Autodesk Inventor part; units mm, degrees
ref_plane "YZ Plane" through (0, 0, 0) normal (1, 0, 0) x (0, 1, 0)
ref_plane "XY Plane" through (0, 0, 0) normal (0, 0, 1) x (1, 0, 0)
sketch "スケッチ1" plane through (0, 0, 0) normal (0, 1, 0) x (-1, 0, 0)
  line L0 (6.5, -6.5) -> (-6.5, -6.5)
  line L1 (-6.5, -6.5) -> (-6.5, 6.5)
  line L2 (-6.5, 6.5) -> (6.5, 6.5)
  line L3 (6.5, 6.5) -> (6.5, -6.5)
  line L4 (6.5, -6.5) -> (-6.5, 6.5) construction
  line L5 (-6.5, -6.5) -> (6.5, 6.5) construction
  dimension "d1" = 13
  dimension "d2" = 13
extrude "押し出し4" add sketch "スケッチ1" along normal blind 5
ref_plane "作業平面2" through (0, 5, 0) normal (0, 1, 0) x (-1, 0, 0)
sketch "スケッチ3" plane through (0, 5, 0) normal (0, 1, 0) x (-1, 0, 0)
  line L0 (4, -4) -> (-4, -4)
  line L1 (-4, -4) -> (-4, 4)
  line L2 (-4, 4) -> (4, 4)
  line L3 (4, 4) -> (4, -4)
  line L4 (4, -4) -> (-4, 4) construction
  line L5 (-4, -4) -> (4, 4) construction
  line L6 (5, -5) -> (-5, -5)
  line L7 (-5, -5) -> (-5, 5)
  line L8 (-5, 5) -> (5, 5)
  line L9 (5, 5) -> (5, -5)
  line L10 (5, -5) -> (-5, 5) construction
  line L11 (-5, -5) -> (5, 5) construction
  point P0 (0, 0)
  point P1 (0, 0)
  dimension "d19" = 8
  dimension "d20" = 8
  dimension "d21" = 10
  dimension "d22" = 10
extrude "押し出し5" cut sketch "スケッチ3" against normal blind 3
hole "穴1" at (0, 5, 0) direction (0, -1, 0) diameter 3.242 end through all
fillet "フィレット1" radius 1 4 edges at (0, 0, -6.5) (6.5, 0, 0) (-6.5, 0, 0) (0, 0, 6.5)
sketch "スケッチ4" plane through (0, 5, 0) normal (0, 1, 0) x (1, 0, 0)
  point P0 (0, 0)
sketch "スケッチ5" plane through (0, 5, 0) normal (0, 1, 0) x (1, 0, 0)
  point P0 (0, 0)
properties part number "pin_joint_ver1"
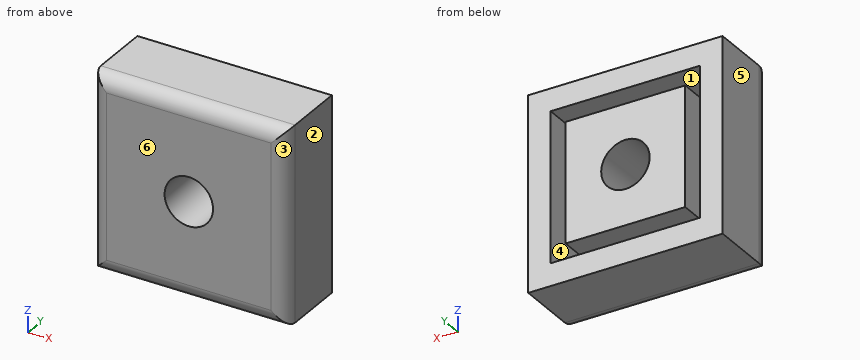
Could you check a few things on this model? Use its own coordinates, in mm. Face numbers are marked on the shaded views. A direction names the side the tool comes from. Give positions to 0.01 mm unless a question says otherwise; leave off trailing zeros. Order: outer loops, then holes, each group sorted by start corner. A loop starts at its lowest first (then second) coordinate and runs counter-clockwise, first axis right, second up. Notation, with made-up numbers: (65, 89.5) -> (104, 89.5) arc R23 cw to (104, 121.5) -> close; hole circle Ø2 at (-24, -9). An arc over 180 degrees is marked (long way). Answer in a Markdown table with one row per item. Add a question column.
Item 1: We'd pull the mould along X, two halves only. Please class the marked faces 3, 4, 5 and 6: pulls with the +X half, pulls with the -X half, needs draft (parallel to the pull), parting line crosses it, or undercut.
Item 2: I'm going to push a flat-ended pin straight in: P1, Ø3, axis at y = 0.5, z = 4, coming from the -X side. Where does the tip first touch, or does it pass through?
Item 3: Please list where these lines run through material, in increasing order: probe 1 along Z at (x, y) = (0, 3.1); probe 2 along X at (y, z) = (3.95, -2.25).
Item 4: Imagine slicing it at D-D (z = 3). List the corners of the cut face in (x, y) for me.
Item 5: Imagine slicing it at A-A (y = 3.4). List the corners of the cut face in (x, z) for me, and give its area (3 significant figures).
Item 6: For the marked faces 1 and 2, which set-ups out of +Z, -Z, +X, -X, +Y, -Y let a thin tool reach every point of the face, with its end or its side?
Item 7: Imagine slicing it at C-C (z = 0). List the corners of the cut face in (x, y) for me.
Item 8: Imagine slicing it at B-B (x = 0). List the corners of the cut face in (y, z) for me.
Result:
| question | item | result |
|---|---|---|
| 1 | face 3 | pulls with the +X half |
| 1 | face 4 | undercut |
| 1 | face 5 | pulls with the -X half |
| 1 | face 6 | needs draft |
| 2 | P1 | x = -6.5 |
| 3 | probe 1 | -6.5 to -5, -4 to -1.62, 1.62 to 4, 5 to 6.5 |
| 3 | probe 2 | -6.5 to -5, -4 to 4, 5 to 6.5 |
| 4 | outline | (-6.5, 1) arc R1 ccw to (-5.5, 0) -> (5.5, 0) arc R1 ccw to (6.5, 1) -> (6.5, 5) -> (5, 5) -> (5, 2) -> (4, 2) -> (4, 5) -> (-4, 5) -> (-4, 2) -> (-5, 2) -> (-5, 5) -> (-6.5, 5) -> close |
| 5 | outline | (-6.5, -6.5) -> (6.5, -6.5) -> (6.5, 6.5) -> (-6.5, 6.5) -> close; (-4, -4) -> (4, -4) -> (4, 4) -> (-4, 4) -> close; hole (-5, -5) -> (5, -5) -> (5, 5) -> (-5, 5) -> close; hole circle Ø3.24 at (0, 0) |
| 5 | area | 125 mm2 |
| 6 | face 1 | +Y |
| 6 | face 2 | +Z, -Z, +X, +Y, -Y |
| 7 | outline | (-6.5, 1) arc R1 ccw to (-5.5, 0) -> (-1.62, 0) -> (-1.62, 5) -> (-4, 5) -> (-4, 2) -> (-5, 2) -> (-5, 5) -> (-6.5, 5) -> close; (1.62, 0) -> (5.5, 0) arc R1 ccw to (6.5, 1) -> (6.5, 5) -> (5, 5) -> (5, 2) -> (4, 2) -> (4, 5) -> (1.62, 5) -> close |
| 8 | outline | (0, -5.5) arc R1 ccw to (1, -6.5) -> (5, -6.5) -> (5, -5) -> (2, -5) -> (2, -4) -> (5, -4) -> (5, -1.62) -> (0, -1.62) -> close; (0, 1.62) -> (5, 1.62) -> (5, 4) -> (2, 4) -> (2, 5) -> (5, 5) -> (5, 6.5) -> (1, 6.5) arc R1 ccw to (0, 5.5) -> close |
